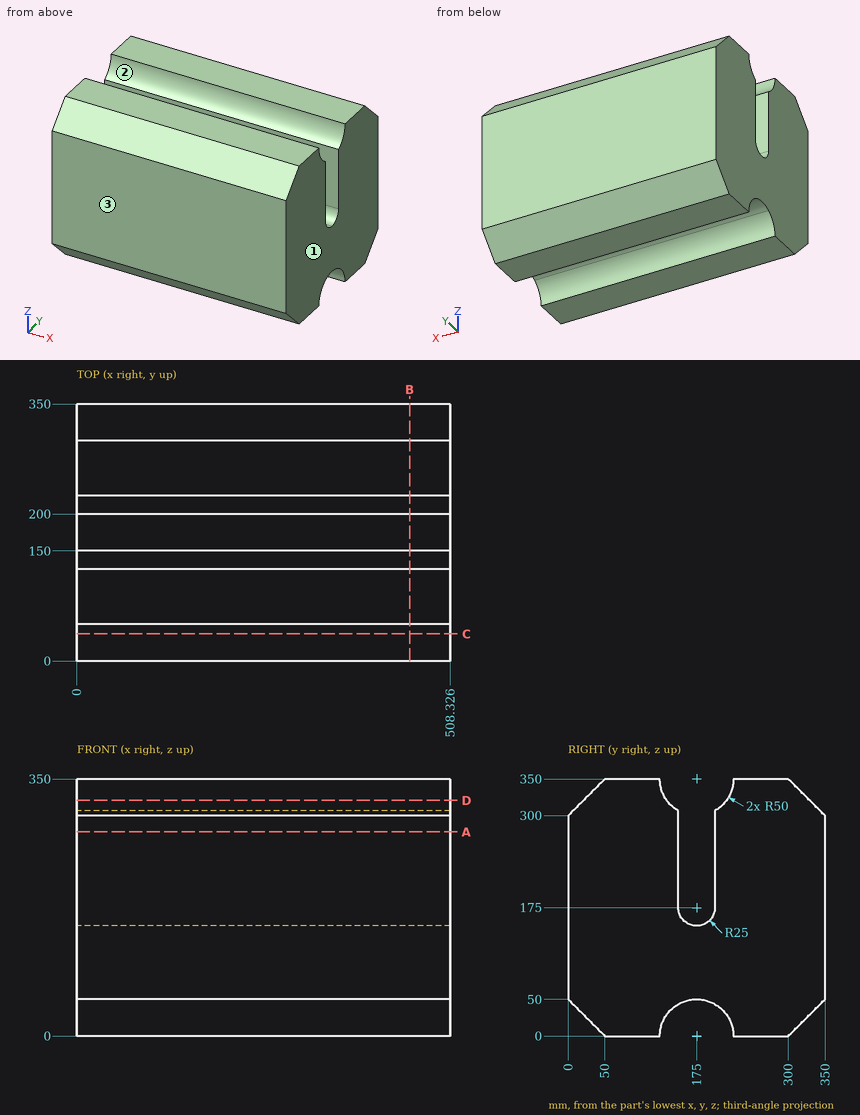
Geometry: see drawing. Coordinates: mm, zero at the bounding-box minimum. Give positions to 0.01 mm unless a question says otherwise; leave off trailing zeros. Order: outer loops, then holes, each group sorted by start corner. A loop starts at its lowest first (then second) coordinate and runs counter-clockwise, first axis right, second up.
Q1. Section D-D on z = 321. Output: boundary loops of the cut face in (x, y), and give its area (3 significant figures).
Checked values:
outline: (0, 21) - (508.33, 21) - (508.33, 134.27) - (0, 134.27) - close; (0, 215.73) - (508.33, 215.73) - (508.33, 329) - (0, 329) - close
area: 115,000 mm2
Q2. Section A-A on z = 278. Output: boundary loops of the cut face in (x, y).
Checked values:
outline: (0, 0) - (508.33, 0) - (508.33, 150) - (0, 150) - close; (0, 200) - (508.33, 200) - (508.33, 350) - (0, 350) - close
Q3. Section B-B on x = 453. Output: boundary loops of the cut face in (y, z).
Checked values:
outline: (0, 50) - (50, 0) - (125, 0) arc R50 cw to (225, 0) - (300, 0) - (350, 50) - (350, 300) - (300, 350) - (225, 350) arc R50 cw to (200, 306.7) - (200, 175) arc R25 cw to (150, 175) - (150, 306.7) arc R50 cw to (125, 350) - (50, 350) - (0, 300) - close
Q4. Ray query, probe 1 along Y at (x, z) = (309, 259); probe 2 along Y at (x, z) = (94, 44.5) (1 decimal); probe 3 along Z at (x, y) = (292.5, 38.5). Return the intervals inside material, ascending.
Checked values:
probe 1: y = 0 to 150, 200 to 350
probe 2: y = 5.5 to 152.2, 197.8 to 344.5
probe 3: z = 11.5 to 338.5
Q5. Section C-C on y = 37. Output: boundary loops of the cut face in (x, z).
Checked values:
outline: (0, 13) - (508.33, 13) - (508.33, 337) - (0, 337) - close
Q6. Draft query along Y for the marked faces 1, 2 and 3. Return one class per face: +Y half, -Y half, draft (parallel to the pull), parting line (faces both ways), or undercut.
Checked values:
face 1: draft
face 2: undercut
face 3: -Y half
